from build123d import *

# Parameters (mm, degrees)
SKETCH1_R           = 3.75
BOSS_EXTRUDE1_DEPTH = 105
SKETCH3_R           = 7.5
BOSS_EXTRUDE2_DEPTH = 2
BOSS_EXTRUDE3_START = 2
SKETCH4_R           = 7.5
BOSS_EXTRUDE3_DEPTH = 2
FILLET1_R           = 5


with BuildPart() as part:
    # Sketch1 → Boss-Extrude1 (new body)
    with BuildSketch(Plane.XY):
        Circle(SKETCH1_R)
    extrude(amount=BOSS_EXTRUDE1_DEPTH)

    # Sketch3 → Boss-Extrude2 (add)
    with BuildSketch(Plane.XY.offset(105)):
        Circle(SKETCH3_R)
    extrude(amount=BOSS_EXTRUDE2_DEPTH)

    # Sketch4 → Boss-Extrude3 (add)
    with BuildSketch(Plane(origin=(0, 0, 0), x_dir=(-1, 0, 0), z_dir=(0, 0, -1)).offset(BOSS_EXTRUDE3_START)):
        with Locations(Location((0, 0, 0), (0, 0, 180))):
            Circle(SKETCH4_R)
    extrude(amount=-BOSS_EXTRUDE3_DEPTH)

    # Fillet1
    # the kernel refuses this fillet: 5 mm, written as the material it takes off along each edge
    with BuildSketch(Plane(origin=(0, 0, -2), x_dir=(1, 0, 0), z_dir=(0, 1, 0))) as fillet1_piece_1:
        with BuildLine():
            CenterArc((3.5, -5), FILLET1_R, 36.869897646, 53.130102354)
            Line((3.5, 0), (3.5, 0.1))
            Line((3.5, 0.1), (7.5, 0.1))
            Line((7.5, 0.1), (7.6, 0))
            ThreePointArc((7.6, 0), (7.6, -1), (7.58, -1.94))
            Line((7.58, -1.94), (7.5, -2))
        make_face()
    revolve(axis=Axis((0, 0, -2), (0, 0, -1)), mode=Mode.SUBTRACT)
    with BuildSketch(Plane(origin=(0, 0, 107), x_dir=(1, 0, 0), z_dir=(0, -1, 0))) as fillet1_piece_2:
        with BuildLine():
            CenterArc((3.5, -5), FILLET1_R, 36.869897646, 53.130102354)
            Line((3.5, 0), (3.5, 0.1))
            Line((3.5, 0.1), (7.5, 0.1))
            Line((7.5, 0.1), (7.6, 0))
            ThreePointArc((7.6, 0), (7.6, -1), (7.58, -1.94))
            Line((7.58, -1.94), (7.5, -2))
        make_face()
    revolve(axis=Axis((0, 0, 107), (0, 0, 1)), mode=Mode.SUBTRACT)


solid = part.part
Input: part model. Units: mm. Frame: model coordinates. Round coordinates to 2 decimals unless told otherwise and drop trailing zeros. Loops run counter-clockwise (first coordinate to the right, second up) from the corner with the lowest first, then second, coordinate; pieces in that order, holes last. Notation, with made-up numbers: M -11,75.25 L 13,75.25 A10 cw 13,87.25 Z; hole C 18,88.5 d8. An arc over 180 degrees is marked long. Answer as CSV lines item,"result". Start each with the question number.
(1) Draft query along Z for faces 1 (the flat face through (0, 0, 107)), 2 (the flat face through (3, 3, 0)), 3 (the flat face through (0, 0, -2)). Return one class per face: released by +Z, released by -Z, zero draft, split by the parting line, or undercut.
(2) First-contact query: pin 1 (3 mm diameter, centred on x = 5, y = 5.5, fed in from -Z); pin 2 (4 mm diameter, centred on y = -4.5, z = 84, fed in from -X); pin 3 (6 mm diameter, centred on x = -0.5, z = 51.5, fed in from +Y). Flat tips, straight axial feed; report the tip coordinate or a pass-through.
(3) Section A-A, the plane z = 62.5. Output: boundary loops of the cut face in (x, y), plus the area to 3 significant figures.
(4) Line query: line 1 (Z direction, x = 3, y = 4); line 2 (Z direction, x = 4.75, y = 5); line 3 (Y direction, x = 0, z = 57.5). Output: solid intervals per line, ascending. Write a range as [from, to].
Values found:
1,face 1,"released by +Z"
1,face 2,"undercut"
1,face 3,"released by -Z"
2,pin 1,"stops at z = -1.37"
2,pin 2,"stops at x = -2.8"
2,pin 3,"stops at y = 3.75"
3,outline,"C 0,0 d7.5"
3,area,"44.2 mm²"
4,line 1,"z = [-1.77, 0], [105, 106.77]"
4,line 2,"z = [-0.67, 0], [105, 105.67]"
4,line 3,"y = [-3.75, 3.75]"
